Part print with two shaded views. Sizes in mm from the minimum x, y, z corner. Round coordinates to 2 decimals unless told otherwise and drop trailing zeros. Write each loop counter-clockwise with the first axis right and the second up, starting at its lowest first coordinate (ties: lowest second). Pieces come first, ordered by that corner, then holes. Notation, with made-up numbers: (41, 39.5) - (97, 39.5) arc R25 cw to (97, 74.5) - close; hole circle Ø2 at (74, 16.5). An arc over 180 degrees is marked (long way). Answer as a JSON object with one key per item and string values. Group by question number.
Item 1: Probe line 1 (Y direction, x = 0.3, z = 5); line 2 (X direction, y = 81, z = 18.5); line 3 (Z direction, x = 9.25, y = 37). List the from-to ranges inside material, lowest first. Write a range as from..to.
Item 2: Slice it at C-C, the plane y = 79.5. List the corners of the cut face in (x, z), then the cut area to 4 significant figures.
Item 3: Slice it at D-D, the plane x = 6. List the corners of the cut face in (y, z), then the cut area to 4 significant figures.
Item 4: Slice it at A-A, the plane z = 5. List the corners of the cut face in (x, y).
Item 5: Two-plate mould, pull along Z, no slides. Class the marked faces 1, 2 and 3: +Z half, -Z half, draft (parallel to the pull), parting line (faces both ways), or undercut.
Item 6: Flat gauge pins, fed straight in: pin 1 (2 mm diameter, centred on y = 28.5, z = 11.5, fed in from +X); pin 2 (6 mm diameter, centred on x = 13, y = 111, fed in from -Z). Where does each tip first touch, or does it go through?
Item 7: Slice it at B-B, the plane y = 110. List the corners of the cut face in (x, z), then the cut area to 3 significant figures.
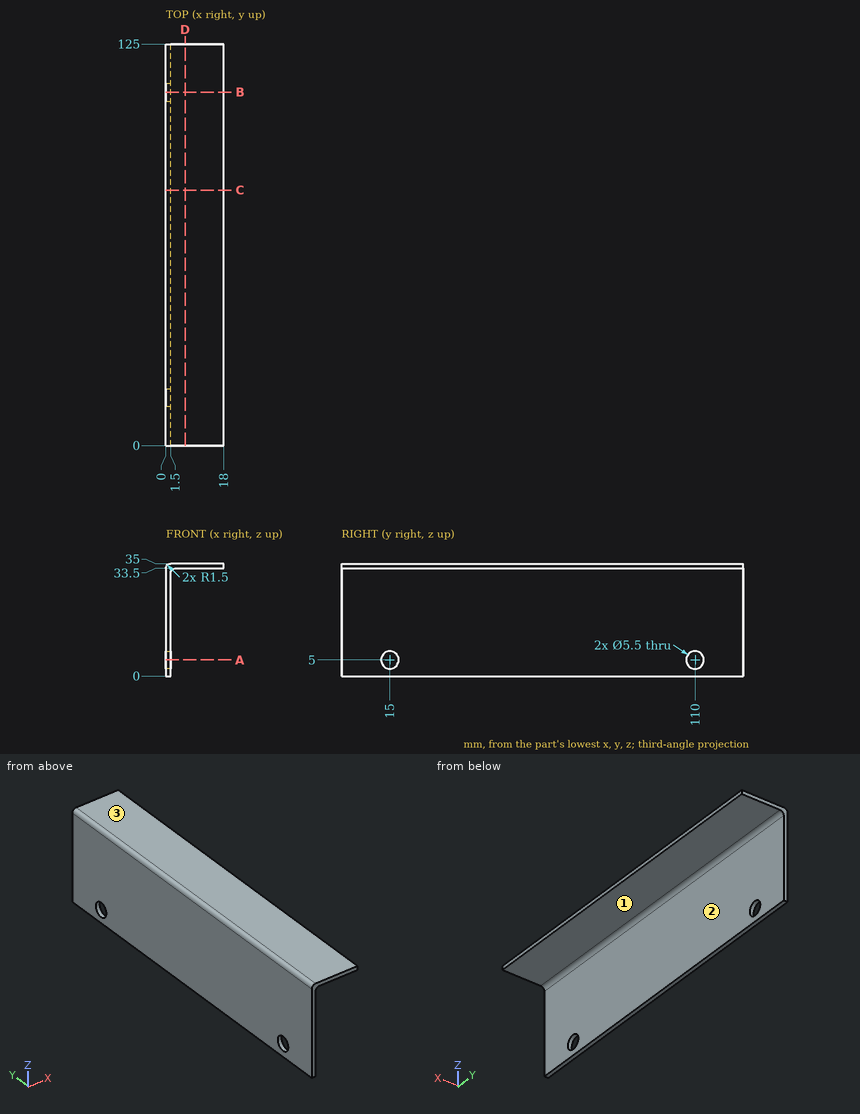
Geometry says:
{
 "1": {"line 1": "y = 0..12.25, 17.75..107.25, 112.75..125", "line 2": "x = 0..1.5", "line 3": "z = 33.5..35"},
 "2": {"outline": "(0, 0) - (1.5, 0) - (1.5, 32) arc R1.5 cw to (3, 33.5) - (18, 33.5) - (18, 35) - (1.5, 35) arc R1.5 ccw to (0, 33.5) - close", "area": "77.25 mm^2"},
 "3": {"outline": "(0, 33.5) - (125, 33.5) - (125, 35) - (0, 35) - close", "area": "187.5 mm^2"},
 "4": {"outline": "(0, 0) - (1.5, 0) - (1.5, 12.25) - (0, 12.25) - close; (0, 17.75) - (1.5, 17.75) - (1.5, 107.25) - (0, 107.25) - close; (0, 112.75) - (1.5, 112.75) - (1.5, 125) - (0, 125) - close"},
 "5": {"face 1": "-Z half", "face 2": "draft", "face 3": "+Z half"},
 "6": {"pin 1": "stops at x = 1.5", "pin 2": "stops at z = 33.5"},
 "7": {"outline": "(0, 0) - (1.5, 0) - (1.5, 2.25) - (0, 2.25) - close; (0, 7.75) - (1.5, 7.75) - (1.5, 32) arc R1.5 cw to (3, 33.5) - (18, 33.5) - (18, 35) - (1.5, 35) arc R1.5 ccw to (0, 33.5) - close", "area": "69.0 mm^2"}
}
